Build history of the part. All positions in model axes, mm. A direction names the side the tool comes from. Round coordinates to 2 decimals unless told otherwise and drop trailing zeros. Loops run counter-clockwise (first coordinate to the right, second up) from the corner with the lowest first, then second, coordinate; pieces in that order, holes last. Notation, with made-up numbers: (60, 10) - (84, 10) arc R17 ccw to (84, 41) - close; hole circle Ø8 at (31, 66.5). An arc over 180 degrees is marked (long way). Use a Markdown table: item, result.
from build123d import *

# Parameters (mm, degrees)
F0_W            = 17
F0_H            = 38
F1_DEPTH        = 3
F2_W            = 17
F2_H            = 5
F3_DEPTH        = 24
F4_R            = 8.49999
F5_R            = 3
F6_DEPTH        = 40
F7_W            = 11
F7_H            = 29.9753743202
F8_DEPTH        = 1
F10_DEPTH       = 2
F11_R           = 5.5
F12_DEPTH       = 1
F14_D           = 1
F14_DEPTH       = 20
F14_TIP         = 0.3004303095
F16_D           = 3
F16_DEPTH       = 20
F16_CBORE_D     = 6.5
F16_CBORE_DEPTH = 1
F16_TIP         = 0.9012909285
F18_R           = 3.5
F19_DEPTH       = 25
F21_DEPTH       = 2
F22_D           = 3


# Not quite as in the source:
# - a fillet or chamfer is up to 0.001 mm smaller than in the source, because OpenCascade refuses the exact size
# - a feature names something its author has since deleted; it is built from what else it names


with BuildPart() as f1:
    # F0 (on Front) → F1 (new body)
    with BuildSketch(Plane.XZ):
        Rectangle(F0_W, F0_H)
    extrude(amount=F1_DEPTH)

    # F2 (on face) → F3 (join)
    with BuildSketch(Plane.XZ.offset(3)):
        with Locations((0, -16.5)):
            Rectangle(F2_W, F2_H)
        with Locations((0, 16.5)):
            Rectangle(F2_W, F2_H)
    extrude(amount=F3_DEPTH)

    # F4 (radius 8.5 in the source; OpenCascade refuses exactly that, so slightly less here)
    f4_edges = [f1.edges().sort_by_distance(p)[0] for p in [
        (8.5, -27, -16.5),
        (-8.5, -27, -16.5),
        (8.5, -27, 16.5),
        (-8.5, -27, 16.5),
    ]]
    fillet(f4_edges, radius=F4_R)

    # F5 (on face) → F6 (cut)
    with BuildSketch(Plane(origin=(0, 0, -19), x_dir=(1, 0, 0), z_dir=(0, 0, -1))):
        with Locations((0, 19)):
            Circle(F5_R)
    extrude(amount=-F6_DEPTH, mode=Mode.SUBTRACT)

    # F7 (on face) → F8 (cut)
    with BuildSketch(Plane.XY.offset(19)):
        with Locations((0, -17.9876871601)):
            Rectangle(F7_W, F7_H)
    extrude(amount=-F8_DEPTH, mode=Mode.SUBTRACT)

    # F9 (on face) → F10 (cut)
    with BuildSketch(Plane(origin=(0, 0, -19), x_dir=(1, 0, 0), z_dir=(0, 0, -1))):
        with BuildLine():
            Line((4.2340652424, 28.3797578726), (-4.2340652424, 28.3797578726))
            Line((-4.2340652424, 28.3797578726), (-3.4896296074, 18.730769238))
            ThreePointArc((-3.4896296074, 18.730769238), (-0.1347152072, 22.4974064409), (3.5, 19))
            ThreePointArc((3.5, 19), (3.4974064409, 18.8652847928), (3.4896296074, 18.730769238))
            Line((3.4896296074, 18.730769238), (4.2340652424, 28.3797578726))
        make_face()
        with BuildLine():
            ThreePointArc((3.4896296074, 18.730769238), (0, 15.5), (-3.4896296074, 18.730769238))
            Line((-3.4896296074, 18.730769238), (-2.4925925763, 5.8076923077))
            ThreePointArc((-2.4925925763, 5.8076923077), (0, 3.5), (2.4925925763, 5.8076923077))
            Line((2.4925925763, 5.8076923077), (3.4896296074, 18.730769238))
        make_face()
        with BuildLine():
            ThreePointArc((3.5, 19), (-0.1347152072, 22.4974064409), (-3.4896296074, 18.730769238))
            ThreePointArc((-3.4896296074, 18.730769238), (0, 15.5), (3.4896296074, 18.730769238))
            ThreePointArc((3.4896296074, 18.730769238), (3.4974064409, 18.8652847928), (3.5, 19))
        make_face()
    extrude(amount=-F10_DEPTH, mode=Mode.SUBTRACT)

    # F11 (on face) → F12 (cut)
    with BuildSketch(Plane(origin=(0, 0, 14), x_dir=(1, 0, 0), z_dir=(0, 0, -1))):
        with Locations((0, 19)):
            Circle(F11_R)
    extrude(amount=-F12_DEPTH, mode=Mode.SUBTRACT)

    # F14
    with Locations(Plane(origin=(0, 0, 0), x_dir=(-1, 0, 0), z_dir=(0, 1, 0))):
        with Locations((-4, 4), (-4, -4)):
            Hole(F14_D / 2, depth=F14_DEPTH)
            with Locations((0, 0, -(F14_DEPTH + F14_TIP / 2))):  # 118° drill point
                Cone(0, F14_D / 2, F14_TIP, mode=Mode.SUBTRACT)

    # F16
    with Locations(Plane.XZ.offset(3)):
        with Locations((4, 4), (4, -4)):
            CounterBoreHole(F16_D / 2, F16_CBORE_D / 2, F16_CBORE_DEPTH, depth=F16_DEPTH)
            with Locations((0, 0, -(F16_DEPTH + F16_TIP / 2))):  # 118° drill point
                Cone(0, F16_D / 2, F16_TIP, mode=Mode.SUBTRACT)

    # F18 (on face) → F19 (cut)
    with BuildSketch(Plane(origin=(0, 0, -17), x_dir=(1, 0, 0), z_dir=(0, 0, -1))):
        with Locations((0, 19)):
            Circle(F18_R)
    extrude(amount=-F19_DEPTH, mode=Mode.SUBTRACT)

    # F20 (on face) → F21 (cut)
    with BuildSketch(Plane.XZ.offset(3)):
        Polygon((-1.2190877389, 5.5914901538), (-3.9878147725, 7.2040857407), (-6.7687270336, 5.6125955869), (-6.7809122611, 2.4085098462), (-4.0121852275, 0.7959142593), (-1.2312729664, 2.3874044131), align=None)
        Polygon((-1.2179301405, -2.4078473634), (-3.9878097002, -0.7945805083), (-6.7698795597, -2.3867331448), (-6.7820698595, -5.5921526366), (-4.0121902998, -7.2054194917), (-1.2301204403, -5.6132668552), align=None)
    extrude(amount=-F21_DEPTH, mode=Mode.SUBTRACT)

    # F22 (through all)
    with Locations(Plane.XZ.offset(3)):
        with Locations((-4, 4), (-4, -4)):
            Hole(F22_D / 2)


solid = f1.part
Q1. Which spindle directions (+Z, -Z, +X, -X, +Y, -Y) get a long thin tool onto all of the face, cutting with end or side? Do faces 1 (the face through (-5.36, -2.01, -1.58)), 2 (the face through (2.4, -16.6, 15)), 3 (the face through (0, -12, 14)), 4 (the face through (-0.1, -3.5, -18)). Say none if no direction does.
Results found:
| item | result |
|---|---|
| face 1 | -Y |
| face 2 | none |
| face 3 | +X, -X, -Y |
| face 4 | -Z, -Y |
Q2. Cut at B-B, the plane y = -21.5. List the corners of the cut face in (x, z), plus the area to 3 significant figures.
Results found:
| item | result |
|---|---|
| outline | (-7.95, -19) - (-3.7, -19) - (-3.7, -17) - (-2.45, -17) - (-2.45, -14) - (-7.95, -14) - close; (-7.95, 14) - (-4.9, 14) - (-4.9, 15) - (-1.66, 15) - (-1.66, 18) - (-5.5, 18) - (-5.5, 19) - (-7.95, 19) - close; (1.66, 15) - (4.9, 15) - (4.9, 14) - (7.95, 14) - (7.95, 19) - (5.5, 19) - (5.5, 18) - (1.66, 18) - close; (2.45, -17) - (3.7, -17) - (3.7, -19) - (7.95, -19) - (7.95, -14) - (2.45, -14) - close |
| area | 98.8 mm2 |
Q3. Cut at D-D, the plane y = -2.5. List the corners of the cut face in (x, z).
Results found:
| item | result |
|---|---|
| outline | (-8.5, -19) - (8.5, -19) - (8.5, 19) - (-8.5, 19) - close; hole (-6.78, -5.59) - (-4.01, -7.21) - (-1.23, -5.61) - (-1.22, -2.41) - (-3.99, -0.79) - (-6.77, -2.39) - close; hole (-6.78, 2.41) - (-4.01, 0.8) - (-1.23, 2.39) - (-1.22, 5.59) - (-3.99, 7.2) - (-6.77, 5.61) - close; hole circle Ø6.5 at (4, -4); hole circle Ø6.5 at (4, 4) |
Q4. Drop flat-ended pins along their axis: pin 1 (4 mm diameter, centred on x = 4, z = -4, fed in from -Y); pin 2 (0.5 mm diameter, centred on x = 0.5, z = 18.5, fed in from -Y); pin 3 (5.5 mm diameter, centred on x = 2, y = -16.5, fed in from +Z). Give the stop position or say it passes through.
Results found:
| item | result |
|---|---|
| pin 1 | stops at y = -2 |
| pin 2 | stops at y = -3 |
| pin 3 | stops at z = 18 |
Q5. Probe line 1 (Z direction, x = -4, y = -0.45); line 2 (Z direction, x = 2.5, y = -24.5); line 3 (Z direction, x = 3.25, y = -5.5). List the from-to ranges inside material, lowest first.
Results found:
| item | result |
|---|---|
| line 1 | z = -19 to -5.5, -2.5 to 2.5, 5.5 to 19 |
| line 2 | z = -17 to -14, 14 to 18 |
| line 3 | z = -19 to -14, 14 to 18 |
Q6. Pull direction Z, two halves, no side cores. Call faces 5 (the face through (-6, -10, 19)), 6 (the face through (-0.65, -16.07, 16.48)), 7 (the face through (-5.43, -0.49, 4.45)): pulls with the +Z half, pulls with the -Z half, needs draft (parallel to the pull), parting line crosses it, or undercut.
Results found:
| item | result |
|---|---|
| face 5 | pulls with the +Z half |
| face 6 | needs draft |
| face 7 | undercut |
Q7. Cut at C-C, the plane z = 4. List the corners of the cut face in (x, y).
Results found:
| item | result |
|---|---|
| outline | (-8.5, -3) - (-6.77, -3) - (-6.77, -1) - (-5.5, -1) - (-5.5, 0) - (-8.5, 0) - close; (-2.5, -1) - (-1.23, -1) - (-1.23, -3) - (0.75, -3) - (0.75, -2) - (2.5, -2) - (2.5, 0) - (-2.5, 0) - close; (5.5, -2) - (7.25, -2) - (7.25, -3) - (8.5, -3) - (8.5, 0) - (5.5, 0) - close |
